Design review of the part built by this model. Coordinates are the model's own, in mm. A direction names the side the tool comes from. Give positions to 0.01 mm unless a question says otherwise; leave off trailing zeros. Write each loop counter-clockwise with the first axis right and the second up, starting at its lowest first coordinate (ties: lowest second). Pieces come first, ordered by that corner, then holes. Notation, with made-up numbers: M 78.5,30 L 119.5,30 A20 ccw 119.5,45 Z; hole C 34.25,79.25 d10. An arc over 180 degrees is marked long. Use one line per item in the form item = value. Start each with the question number.
from build123d import *

# Parameters (mm, degrees)
SKETCH_1_W               = 25
SKETCH_1_H               = 25
SKETCH_1_W_2             = 19
SKETCH_1_H_2             = 19
EXTRUDE_1_DEPTH          = 280
SKETCH_2_R               = 3
CUT_EXTRUDE_1_DEPTH      = 283.223315833
CUT_EXTRUDE_2_DEPTH      = 283.223315833
CUT_EXTRUDE_2_DEPTH_BACK = 283.223315833
SKETCH_3_R               = 1.5


with BuildPart() as part:
    # 草图1 → 凸台-拉伸1 (new body)
    with BuildSketch(Plane(origin=(0, 0, 0), x_dir=(1, 0, 0), z_dir=(0, 1, 0))):
        with Locations((12.5, 12.5)):
            Rectangle(SKETCH_1_W, SKETCH_1_H)
        with Locations((12.5, 12.5)):
            Rectangle(SKETCH_1_W_2, SKETCH_1_H_2, mode=Mode.SUBTRACT)
    extrude(amount=EXTRUDE_1_DEPTH)

    # 草图2 → 切除-拉伸1 (cut, through all)
    with BuildSketch(Plane(origin=(0, 0, 0), x_dir=(0, 0, -1), z_dir=(1, 0, 0))):
        with Locations(Location((12.5, 10, 0), (0, 0, 180))):
            Circle(SKETCH_2_R)
        with Locations(Location((12.5, 40, 0), (0, 0, 180))):
            Circle(SKETCH_2_R)
        with Locations(Location((12.5, 70, 0), (0, 0, 180))):
            Circle(SKETCH_2_R)
        with Locations(Location((13, 140, 0), (0, 0, 180))):
            Circle(SKETCH_2_R)
    extrude(amount=CUT_EXTRUDE_1_DEPTH, mode=Mode.SUBTRACT)

    # 草图3 → 切除-拉伸2 (cut, two sides: drawn at the far end of the back side and taken through both)
    with BuildSketch(Plane.XY.offset(-CUT_EXTRUDE_2_DEPTH_BACK)):
        with Locations((6, 180)):
            Circle(SKETCH_3_R)
        with Locations((6, 215)):
            Circle(SKETCH_3_R)
    extrude(amount=CUT_EXTRUDE_2_DEPTH + CUT_EXTRUDE_2_DEPTH_BACK, mode=Mode.SUBTRACT)


solid = part.part
1. To check wall thickness, follow L1, parallel to Y at x = 6, z = -23.1; L2, parallel to Z at x = 20.75, y = 21; L3, parallel to Y at x = 23, z = -12.5. State the ranges of each line that lie inside material, in increasing order.
2. Draft analysis for pull direction Z (two halves, no side actions). For faces 1 (the cylindrical face through (23.48, 72.93, -13.15)), 2 (the flat face through (0, 138, -10)), 3 (the flat face through (12, 138, 0)), state which applies: pulls with the +Z half, pulls with the -Z half, needs draft (parallel to the pull), parting line crosses it, or undercut.
3. We need section D-D (y = 85.5). State the section outline as (x, z) points, and give its area (3 significant figures).
4. We need section B-B (x = 10.75). State the section outline as (y, z) points.
5. We need section C-C (z = -18.5). State the section outline as (x, y) points.
6. For faces 4 (the flat face through (12, 138, -3)), 5 (the flat face through (23, 0, -13)), list the 3-axis set-ups (+Z, -Z, +X, -X, +Y, -Y) from which the entire face can be reached by the end or side of a thin tool; tool diameter is ignored.
7. We need section A-A (y = 140). State the section outline as (x, z) points, and give its area (3 significant figures).
Answer block:
q1.L1 = 0 to 178.5, 181.5 to 213.5, 216.5 to 280
q1.L2 = -25 to -22, -3 to 0
q1.L3 = 0 to 7, 13 to 37, 43 to 67, 73 to 137.04, 142.96 to 280
q2.face_1 = undercut
q2.face_2 = needs draft
q2.face_3 = pulls with the +Z half
q3.outline = M 0,-25 L 25,-25 L 25,0 L 0,0 Z; hole M 3,-22 L 22,-22 L 22,-3 L 3,-3 Z
q3.area = 264 mm^2
q4.outline = M 0,-25 L 280,-25 L 280,-22 L 0,-22 Z; M 0,-3 L 280,-3 L 280,0 L 0,0 Z
q5.outline = M 0,0 L 3,0 L 3,280 L 0,280 Z; M 22,0 L 25,0 L 25,280 L 22,280 Z
q6.face_4 = +Y, -Y
q6.face_5 = +Z, -Z, +X, -X, -Y
q7.outline = M 0,-25 L 25,-25 L 25,-16 L 22,-16 L 22,-22 L 3,-22 L 3,-16 L 0,-16 Z; M 0,-10 L 3,-10 L 3,-3 L 22,-3 L 22,-10 L 25,-10 L 25,0 L 0,0 Z
q7.area = 228 mm^2
